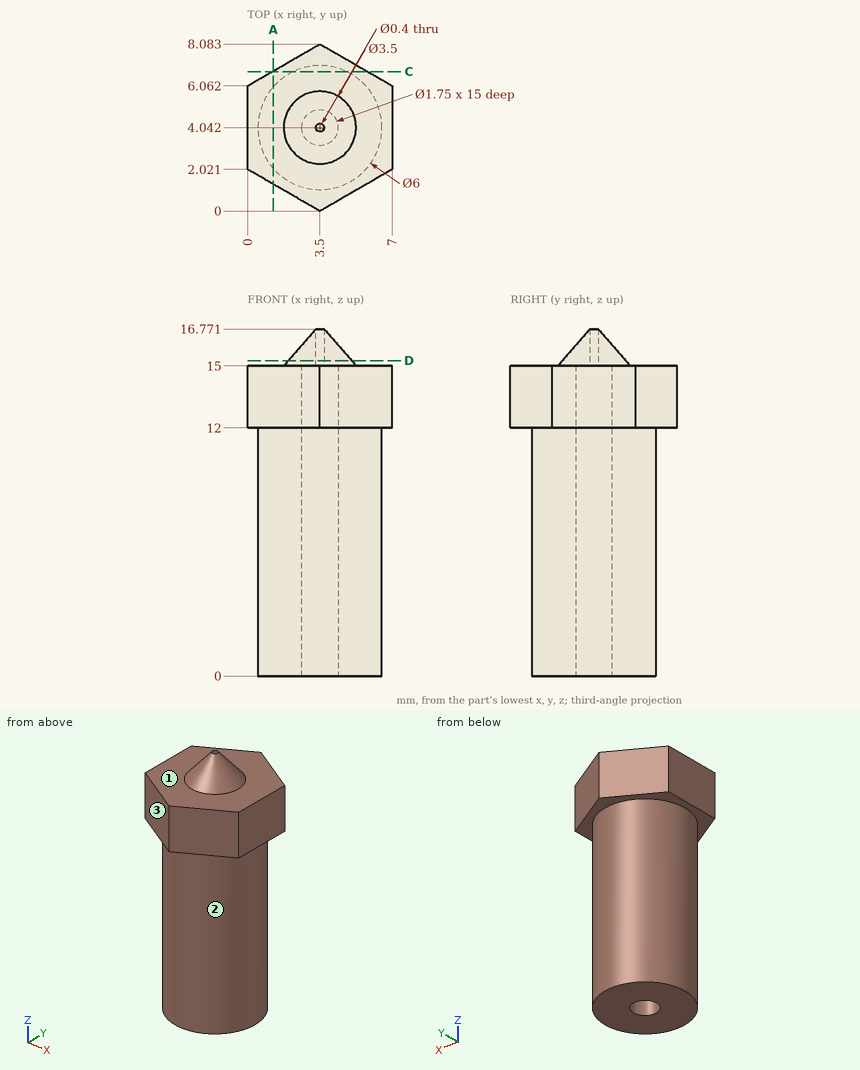
Input: dimensioned drawing with shaded views. Units: mm. Origin: part minimum x, y, z. A direction names the side the tool comes from. Coordinates: 2 decimals unless noted, no trailing zeros. Loops run counter-clockwise (first coordinate to the right, second up) from the corner with the lowest first, then second, coordinate; pieces in that order, holes last. Notation, with made-up numbers: (67, 32) - (75, 32) arc R14 cw to (75, 56) - close; hole circle Ø9 at (77.25, -33). An arc over 180 degrees is marked (long way). One line per question, with ' | ' between items. Start each with the question number.
(1) Cut plane D-D on z = 15.25. Output: boundary loops of the cut face in (x, y).
(2) Cut plane C-C on y = 6.75. Output: boundary loops of the cut face in (x, z).
(3) Ray query, L1, parallel to Y at x = 3.5, z = 10; L2, parallel to Z at x = 1, y = 3.5; L3, parallel to X at y = 3.75, z = 11.5 (1 decimal). Return the intervals inside material, ascending. Write a range as from..to.
(4) First-contact query: pin 1 (1 mm diameter, centred on x = 0.5, y = 6, fed in from -Z); pin 2 (4 mm diameter, centred on x = 1.5, y = 3, fed in from +Z); pin 3 (4 mm diameter, centred on y = 6.5, z = 7.5, fed in from +X) (1 decimal). Flat tips, straight axial feed; report the tip coordinate or a pass-through.
(5) Cut plane A-A on x = 1.25. Output: boundary loops of the cut face in (y, z) (1 decimal).
(6) Reachability of the marked faces 1, 2 and 3 from +Z, -Z, +X, -X, +Y, -Y: full face, straight path, thin tool, end or side. Return the list, or none.
Here are the results:
1) outline: circle Ø3.06 at (3.5, 4.04); hole circle Ø0.4 at (3.5, 4.04)
2) outline: (1.19, 12) - (2.21, 12) - (2.21, 0) - (4.79, 0) - (4.79, 12) - (5.81, 12) - (5.81, 15) - (1.19, 15) - close
3) L1: 1.04..3.17, 4.92..7.04 | L2: 0..15 | L3: 0.5..2.7, 4.3..6.5
4) pin 1: z = 12 | pin 2: z = 16.71 | pin 3: x = 6.5
5) outline: (1.3, 12) - (2.1, 12) - (2.1, 0) - (6, 0) - (6, 12) - (6.8, 12) - (6.8, 15) - (1.3, 15) - close
6) face 1: +Z | face 2: -Z | face 3: +Z, -Z, -X, -Y
